```python
from build123d import *

# Parameters (mm, degrees)
F0_W     = 700
F0_H     = 270
F1_DEPTH = 5
F3_DEPTH = 25
F4_R     = 4
F5_R     = 2


with BuildPart() as f1:
    # F0 (on Top) → F1 (new body)
    with BuildSketch(Plane.XY):
        Rectangle(F0_W, F0_H)
    extrude(amount=F1_DEPTH)

    # F2 (on face) → F3 (cut)
    with BuildSketch(Plane.XY.offset(5)):
        Polygon((-261.5147186258, 135), (-270, 135), (-199.2893218813, 64.2893218813), (-195.0466811942, 68.5319625685), align=None)
        Polygon((270, 135), (261.5147186258, 135), (195.0466811942, 68.5319625685), (199.2893218813, 64.2893218813), align=None)
    extrude(amount=-F3_DEPTH, mode=Mode.SUBTRACT)

    # F4
    f4_edges = [f1.edges().sort_by_distance(p)[0] for p in [
        (-350, -135, 2.5),
        (350, -135, 2.5),
        (350, 135, 2.5),
        (-350, 135, 2.5),
        (-270, 135, 2.5),
        (270, 135, 2.5),
    ]]
    fillet(f4_edges, radius=F4_R)

    # F5
    f5_edges = [f1.edges().sort_by_distance(p)[0] for p in [
        (261.514719, 135, 2.5),
        (-261.514719, 135, 2.5),
    ]]
    fillet(f5_edges, radius=F5_R)


solid = f1.part
```
Source: CAD feature listing. Evaluate the final solid. Frame: model axes, mm. A direction names the side the tool comes from. Coordinates: 2 decimals unless noted, no trailing zeros. Loops run counter-clockwise (first coordinate to the right, second up) from the corner with the lowest first, then second, coordinate; pieces in that order, holes last. Notation, with made-up numbers: M 71,3.25 L 91,3.25 A20 ccw 91,10.25 Z; hole C 69.5,-7.5 d9. An arc over 180 degrees is marked long. Use a Markdown table: item, result. Add a question column.
Q1. Material intervals for L1, parallel to X at y = 73.5, z = 0.75; L2, parallel to X at y = 117, z = 4.2; L3, parallel to Y at x = 219, z = 2.9, sorted ascending.
Q2. Section query B-B, the plane y = 83. Return loops of the section in (x, z), and give its area (3 significant figures).
Q3. Draft query along Y for faces 1 (the flat face through (234, 99, 3)), 2 (the flat face through (-226.132, 99.617, 2.535)), 3 (the flat face through (-5, 2, 0)). Return one class per face: pulls with the +Y half, pulls with the -Y half, needs draft (parallel to the pull), parting line crosses it, or undercut.
Q4. Access query for faces 4 (the flat face through (-235, 100, 3)), 5 (the flat face through (-5, 2, 5)). Directions: +Z, -Z, +X, -X, +Y, -Y. A direction counts if a zero-diameter tool reaches every point of the face in a straight line with its end or side. Return the directions, or none.
Q5. Section query A-A, the plane x = -238.5. Return loops of the section in (y, z).
Result:
| question | item | result |
|---|---|---|
| 1 | L1 | x = -350 to -208.5, -200.01 to 200.01, 208.5 to 350 |
| 1 | L2 | x = -350 to -252, -243.51 to 243.51, 252 to 350 |
| 1 | L3 | y = -135 to 84, 92.49 to 135 |
| 2 | outline | M -350,0 L -218,0 L -218,5 L -350,5 Z; M -209.51,0 L 209.51,0 L 209.51,5 L -209.51,5 Z; M 218,0 L 350,0 L 350,5 L 218,5 Z |
| 2 | area | 3,420 mm2 |
| 3 | face 1 | undercut |
| 3 | face 2 | undercut |
| 3 | face 3 | needs draft |
| 4 | face 4 | +Z, -Z |
| 4 | face 5 | +Z, +X, -X, +Y, -Y |
| 5 | outline | M -135,0 L 103.5,0 L 103.5,5 L -135,5 Z; M 111.99,0 L 135,0 L 135,5 L 111.99,5 Z |
